Read the model definition and answer for the solid it produces. Units are mm, in the model's axes. Coordinates: 2 decimals unless noted, no trailing zeros. Loops run counter-clockwise (first coordinate to the right, second up) from the corner with the lowest first, then second, coordinate; pieces in that order, holes last. Notation, with made-up numbers: (63, 45) - (96, 45) arc R15 ccw to (96, 52) - close; hole circle Ø8 at (39, 55.5). An arc over 180 degrees is marked (long way). One line per question, with ' | ' between items. Start each with the question number.
Autodesk Inventor part; units mm, degrees
ref_plane "YZ Plane" through (0, 0, 0) normal (1, 0, 0) x (0, 1, 0)
ref_plane "XZ Plane" through (0, 0, 0) normal (0, 1, 0) x (-1, 0, 0)
ref_plane "XY Plane" through (0, 0, 0) normal (0, 0, 1) x (1, 0, 0)
sketch "草圖1" plane through (0, 0, 0) normal (0, 1, 0) x (-1, 0, 0)
  line L0 (-50, 75) -> (50, 75)
  line L1 (50, 75) -> (50, -75)
  line L2 (50, -75) -> (-50, -75)
  line L3 (-50, -75) -> (-50, 75)
  line L4 (-50, 75) -> (50, -75) construction
  line L5 (50, 75) -> (-50, -75) construction
  point P0 (0, 0)
  dimension "d0" = 100
  dimension "d1" = 150
extrude "擠出1" add sketch "草圖1" along normal blind 55
sketch "草圖2" plane through (0, 55, 0) normal (0, 1, 0) x (1, 0, 0)
  circle A0 centre (0, 49.596879) radius 15.361397
  point P0 (0, 0)
extrude "擠出2" add sketch "草圖2" along normal blind 92.5
sketch "草圖3" plane through (0, 147.5, -49.596879) normal (0, 1, 0) x (1, 0, 0)
  circle A0 centre (0, 0) radius 15.361397
  point P0 (0, -49.596879)
extrude "擠出3" add sketch "草圖3" along normal blind 15 draft -30
sketch "草圖8" plane through (0, 162.5, -49.596879) normal (0, 1, 0) x (1, 0, 0)
  circle A0 centre (0, 0) radius 6.701143
  line L0 (0, 0) -> (-74.851571, -205.653002)
  line L1 (0, 0) -> (218.851354, 0) construction
  point P0 (0, -49.596879)
  dimension "d14" = 110
surface extrude "擠出表面2" sketch "草圖8" along normal blind 8 shown no curves L0
sketch "草圖4" plane through (-14.690503, 0, -9.235054) normal (0.9396926, 0, 0.3420201) x (0, 1, 0)
  line L0 (55, -69.985594) -> (0, -69.985594) construction
  line L1 (0, -69.985594) -> (0, 89.641072) construction
  line L2 (55, 89.641072) -> (55, -27.590761) construction
  line L3 (55, -27.590761) -> (147.5, -27.590761) construction
  line L4 (147.5, -27.590761) -> (162.5, -36.251015) construction
  line L5 (162.5, -36.251015) -> (162.5, -49.6533) construction
  line L6 (162.5, -49.6533) -> (147.5, -58.313554) construction
  line L7 (147.5, -58.313554) -> (55, -58.313554) construction
  line L8 (55, -58.313554) -> (55, -69.985594) construction
  line L9 (162.5, -36.251015) -> (162.5, -49.6533) construction
  arc A0 (162.5, -42.952157) -> (266.230331, -3.041729) centre (162.5, 111.804689) ccw
  line L10 (266.230331, -3.041729) -> (563.073853, 265.070045)
  line L11 (0, 89.641072) -> (55, 89.641072)
  point P0 (0, 3.653664)
  dimension "d8" = 400
sketch "草圖5" plane through (0, 162.5, -49.596879) normal (0, 1, 0) x (1, 0, 0)
  circle A0 centre (0, 0) radius 6.701143
  point P0 (0, -49.596879)
sweep "掃掠1" add profiles "草圖5" path "草圖4" path curves A0 L10
sketch "草圖6" plane through (-105.349798, 563.073853, 239.849311) normal (-0.2292491, 0.7421088, 0.6298566) x (0.9554499, 0.2951535, 0)
  circle A0 centre (0, 0) radius 6.701143
  circle A1 centre (0, 0) radius 6.701143
  line L0 (-6.701143, 0) -> (6.701143, 0)
  point P0 (-65.536753, -172.147129)
  point P1 (0, 0)
surface extrude "擠出表面1" sketch "草圖6" along normal blind 8 shown yes curves L0
sketch "草圖7" plane through (-98.947192, 565.051719, 239.849311) normal (-0.1859044, 0.6017964, -0.7767114) x (-0.9554499, -0.2951535, 0)
  line L0 (13.402285, 0) -> (0, 0)
  line L1 (13.402285, 0) -> (0, 0)
  spline S0 degree 4 poles (13.402285, 0) (44.904659, 17.87413) (4.281315, 87.58342) (-27.060021, 18.156606) (0, 0) knots 0 0 0 0 0 1 1 1 1 1
  line L2 (6.701143, 41.850443) -> (6.701143, 0)
  line L3 (13.402285, 0) -> (0, 0)
  point P0 (72.237896, -593.084089)
  point P1 (21.56931, 30.293196)
  point P2 (-7.261182, 30.293196)
revolve "迴轉1" add sketch "草圖7" angle 360 about axis through (-114.943973, 594.131436, 266.20909) along (0.2292491, -0.7421088, -0.6298566) picked at (11.989428, 23.179775) contours L0 L2 S0
properties part number "無線麥克風組"
1) Given pin 1 Ø16.5 at (x, y) = (-21.5, 35) entering from +Z; pin 2 Ø6 at (y, z) = (390, 82.5) entering from +X; pin 3 Ø1 at (x, z) = (1, 75) entering from -Y, each flat-ended and moving along its own axis, determine where each tip first touches the part or whether it passes through.
2) The mould has two halves that part along Y. Classify faces 1 (the flat face through (50, 27, -1)), 2 (the flat face through (1, 0, 1)), 3 (the conical face through (4.411, 159.895, -42.678)): released by +Y, released by -Y, zero draft, split by the parting line, or undercut.
3) The part is cut by section B-B on y = 97.5. Write down the section's boundary in (x, z), and give its area (3 significant figures).
4) Find the intervals of material crossed by line 1 along Z through (x, y) = (-0.5, 116.5); line 2 along Y through (x, z) = (13, 39); line 3 along Z through (x, y) = (-51, 393.5), in increasing order. Write a range as from..to.
5) The part is cut by section A-A on x = 26. Write down the section's boundary in (y, z), and give its area (3 significant figures).
Answer below:
1) pin 1: z = 75 | pin 2: x = -45.6 | pin 3: y = 0
2) face 1: zero draft | face 2: released by -Y | face 3: undercut
3) outline: circle Ø30.72 at (0, -49.6) | area: 741 mm2
4) line 1: -64.95..-34.24 | line 2: 0..55 | line 3: 87.17..103.74
5) outline: (0, -75) - (55, -75) - (55, 75) - (0, 75) - close | area: 8,250 mm2
